from build123d import *

# Parameters (mm, degrees)
SKETCH1_W           = 38
SKETCH1_H           = 30
BOSS_EXTRUDE1_DEPTH = 14
SKETCH2_W           = 38
SKETCH2_H           = 10
BOSS_EXTRUDE2_DEPTH = 38
SKETCH3_R           = 1.01
CUT_EXTRUDE1_DEPTH  = 38
CUT_EXTRUDE2_DEPTH  = 38
SKETCH5_W           = 4
SKETCH5_H           = 10
CUT_EXTRUDE3_DEPTH  = 12
SKETCH6_R           = 1.25
CUT_EXTRUDE4_DEPTH  = 31
SKETCH8_W           = 38
SKETCH8_H           = 5
CUT_EXTRUDE5_DEPTH  = 31


with BuildPart() as part:
    # Sketch1 → Boss-Extrude1 (new body)
    with BuildSketch(Plane(origin=(0, 0, 0), x_dir=(1, 0, 0), z_dir=(0, 1, 0))):
        with Locations((2.714285714, 1.989417989)):
            Rectangle(SKETCH1_W, SKETCH1_H)
    extrude(amount=BOSS_EXTRUDE1_DEPTH)

    # Sketch2 → Boss-Extrude2 (add)
    with BuildSketch(Plane(origin=(0, 14, 0), x_dir=(1, 0, 0), z_dir=(0, 1, 0))):
        with Locations((2.714285714, 1.989417989)):
            Rectangle(SKETCH2_W, SKETCH2_H)
    extrude(amount=BOSS_EXTRUDE2_DEPTH)

    # Sketch3 → Cut-Extrude1 (cut)
    with BuildSketch(Plane(origin=(0, 0, -6.989417989), x_dir=(-1, 0, 0), z_dir=(0, 0, -1))):
        with Locations((-16.654285714, 47.466668182)):
            Circle(SKETCH3_R)
        with Locations((11.225714286, 47.466668182)):
            Circle(SKETCH3_R)
        with Locations((-16.654285714, 19.586668182)):
            Circle(SKETCH3_R)
        with Locations((11.225714286, 19.586668182)):
            Circle(SKETCH3_R)
    extrude(amount=-CUT_EXTRUDE1_DEPTH, mode=Mode.SUBTRACT)

    # Sketch4 → Cut-Extrude2 (cut)
    with BuildSketch(Plane(origin=(0, 0, -6.989417989), x_dir=(-1, 0, 0), z_dir=(0, 0, -1))):
        Polygon((-14.154285714, 47.396812474), (-14.154285714, 50), (8.725714286, 50), (8.725714286, 44.966668182), (14.285714286, 44.966668182), (14.285714286, 22.086668182), (8.725714286, 22.086668182), (8.725714286, 16), (-14.154285714, 16), (-14.154285714, 22.086668182), (-19.714285714, 22.086668182), (-19.714285714, 44.966668182), (-14.154285714, 44.966668182), align=None)
    extrude(amount=-CUT_EXTRUDE2_DEPTH, mode=Mode.SUBTRACT)

    # Sketch5 → Cut-Extrude3 (cut)
    with BuildSketch(Plane.ZY.offset(16.285714286)):
        with Locations((-4.989417989, 29)):
            Rectangle(SKETCH5_W, SKETCH5_H)
    extrude(amount=-CUT_EXTRUDE3_DEPTH, mode=Mode.SUBTRACT)

    # Sketch6 → Cut-Extrude4 (cut)
    with BuildSketch(Plane(origin=(0, 14, 0), x_dir=(1, 0, 0), z_dir=(0, 1, 0))):
        with Locations((-13.285714286, 9.989417989)):
            Circle(SKETCH6_R)
        with Locations((18.714285714, 9.989417989)):
            Circle(SKETCH6_R)
        with Locations((18.714285714, -10.010582011)):
            Circle(SKETCH6_R)
        with Locations((-13.285714286, -10.010582011)):
            Circle(SKETCH6_R)
    extrude(amount=-CUT_EXTRUDE4_DEPTH, mode=Mode.SUBTRACT)

    # Sketch8 → Cut-Extrude5 (cut)
    with BuildSketch(Plane(origin=(0, 14, 0), x_dir=(1, 0, 0), z_dir=(0, 1, 0))):
        with Locations((2.714285714, 14.489417989)):
            Rectangle(SKETCH8_W, SKETCH8_H)
    extrude(amount=-CUT_EXTRUDE5_DEPTH, mode=Mode.SUBTRACT)


solid = part.part
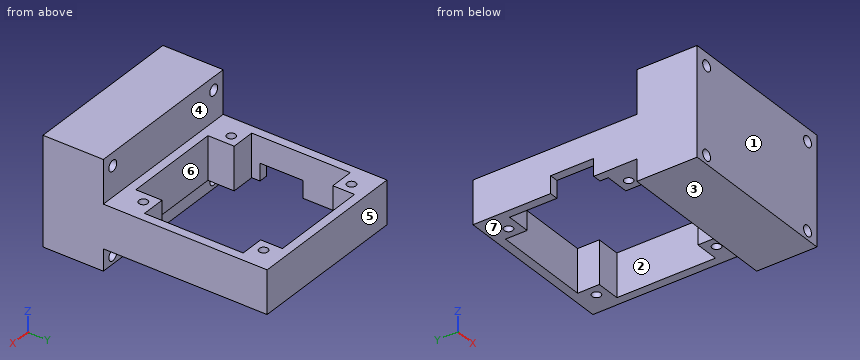
Verification items for the finished model (mm, model axes). Face numbers are marked on the shaded views. A direction names the side the tool comes from. Coordinates: 2 decimals unless noted, no trailing zeros. Loops run counter-clockwise (first coordinate to the right, second up) from the corner with the lowest first, then second, coordinate; pieces in that order, holes last. Notation, with made-up numbers: (7.5, -34.75) -> (30.5, -34.75) arc R35 ccw to (30.5, 2.25) -> close; hole circle Ø1 at (54, -28). An arc over 180 degrees is marked (long way). Answer as a JSON object with one key per item and string values. Group by question number.
Item 1: Depth check by flat-ended pin: pin 1 (2.5 mm diameter, centred on x = 16.65, y = 47.47, fed in from -Z); pin 2 (4 mm diameter, centred on x = -13.29, z = 10.01, fed in from +Y); pin 3 (1.6 mm diameter, centred on x = -15.5, y = 30, fed in from -Z). Enter the tip coordinate at first touch or a pass-through.
Item 2: Sectioned sample at C-C on z = 1. Record the boundary of the cut face in (x, y).
Item 3: Tool access check on the marked faces 4, 5, 6 and 7. Record the directions out of +Z, -Z, +X, -X, +Y, -Y that give a thin tool (end or side, any length) a straight path to the whole face; none if there is none.
Item 4: Sectioned sample at B-B on y = 6. Record the boundary of the cut face in (x, z), plus the area to 3 significant figures.
Item 5: Mould release check, pull along Y, two halves, no side actions. Record for the marked faces 1, 2 and 3: +Y half, -Y half, draft (parallel to the pull), parting line (faces both ways), or undercut.
Item 6: Sectioned sample at D-D on z = -5. Record the boundary of the cut face in (x, y).
Item 7: Scan lines: probe 1 along X at (y, z) = (17.5, -6.75); probe 2 along X at (y, z) = (42, 0.75); probe 3 along Y at (x, z) = (0, -11). Record each from-to range of solid material in increasing order.
Item 8: Sectioned sample at A-A on x = 8. Record the boundary of the cut face in (y, z).
Evaluation:
{
 "1": {"pin 1": "stops at z = -6.99", "pin 2": "stops at y = 14", "pin 3": "stops at z = -2.99"},
 "2": {"outline": "(-16.29, 0) -> (21.71, 0) -> (21.71, 52) -> (-16.29, 52) -> close; hole (-14.29, 22.09) -> (-8.73, 22.09) -> (-8.73, 16) -> (14.15, 16) -> (14.15, 22.09) -> (19.71, 22.09) -> (19.71, 44.97) -> (14.15, 44.97) -> (14.15, 50) -> (-8.73, 50) -> (-8.73, 44.97) -> (-14.29, 44.97) -> close; hole circle Ø2.02 at (-11.23, 19.59); hole circle Ø2.02 at (-11.23, 47.47); hole circle Ø2.02 at (16.65, 19.59); hole circle Ø2.02 at (16.65, 47.47)"},
 "3": {"face 4": "+Z, +X, -X, +Y", "face 5": "+Z, -Z, +X, -X, +Y", "face 6": "+Z, -Z", "face 7": "-Z, +X, -X, +Y"},
 "4": {"outline": "(-16.29, -11.99) -> (21.71, -11.99) -> (21.71, 13.01) -> (-16.29, 13.01) -> close; hole circle Ø2.5 at (-13.29, -9.99); hole circle Ø2.5 at (-13.29, 10.01); hole circle Ø2.5 at (18.71, -9.99); hole circle Ø2.5 at (18.71, 10.01)", "area": "930 mm²"},
 "5": {"face 1": "-Y half", "face 2": "undercut", "face 3": "draft"},
 "6": {"outline": "(-16.29, 0) -> (21.71, 0) -> (21.71, 52) -> (-16.29, 52) -> (-16.29, 34) -> (-14.29, 34) -> (-14.29, 44.97) -> (-8.73, 44.97) -> (-8.73, 50) -> (14.15, 50) -> (14.15, 44.97) -> (19.71, 44.97) -> (19.71, 22.09) -> (14.15, 22.09) -> (14.15, 16) -> (-8.73, 16) -> (-8.73, 22.09) -> (-14.29, 22.09) -> (-14.29, 24) -> (-16.29, 24) -> close; hole circle Ø2.02 at (-11.23, 19.59); hole circle Ø2.02 at (-11.23, 47.47); hole circle Ø2.02 at (16.65, 19.59); hole circle Ø2.02 at (16.65, 47.47)"},
 "7": {"probe 1": "x = -16.29 to -8.73, 14.15 to 21.71", "probe 2": "x = -16.29 to -14.29, 19.71 to 21.71", "probe 3": "y = 0 to 14"},
 "8": {"outline": "(0, -11.99) -> (14, -11.99) -> (14, -6.99) -> (16, -6.99) -> (16, 3.01) -> (14, 3.01) -> (14, 13.01) -> (0, 13.01) -> close; (50, -6.99) -> (52, -6.99) -> (52, 3.01) -> (50, 3.01) -> close"}
}
